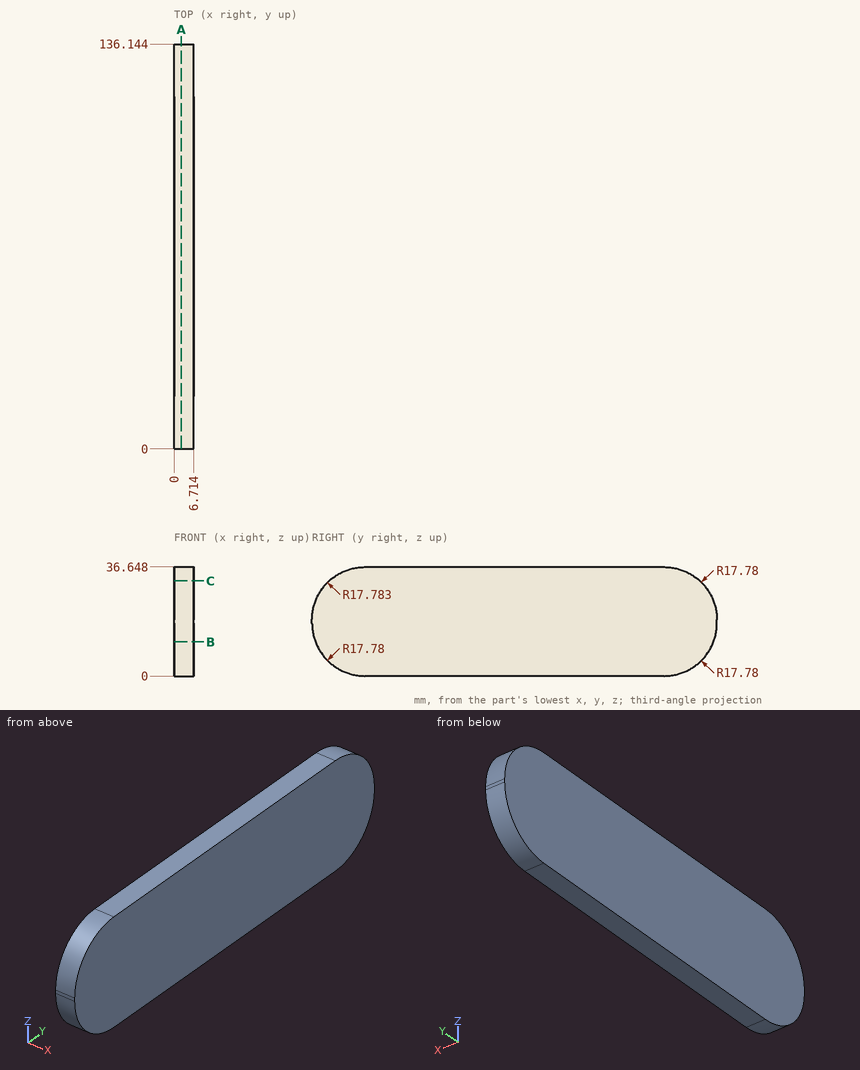
Input: dimensioned drawing with shaded views. Units: mm. Origin: part minimum x, y, z. Round coordinates to 2 decimals unless told otherwise and drop trailing zeros. Loops run counter-clockwise (first coordinate to the right, second up) from the corner with the lowest first, then second, coordinate; pieces in that order, holes last.
1) Pin query (flat end, axial travel): pin 1 (4 mm diameter, centred on x = 6, z = 10, fed in from -Y); pin 2 (1.5 mm diameter, centred on x = 4, z = 6.5, fed in from +Y); pin 3 (3 mm diameter, centred on x = 2, z = 30, fed in from +Y). Return the tip coordinate at first contact, or that it passes through.
Ans:
pin 1: stops at y = 0.97
pin 2: stops at y = 132.69
pin 3: stops at y = 133.31
2) Section query B-B on z = 11.5. Return the cut outline in (x, y), plus the area to 3 significant figures.
Ans:
outline: (0, 1.15) - (6.71, 1.15) - (6.71, 135) - (0, 135) - close
area: 899 mm2
3) Section query A-A on x = 2.5. Return the cut outline in (y, z) (3 decimals).
Ans:
outline: (0, 17.78) arc R17.78 ccw to (17.78, 0) - (118.364, 0) arc R17.78 ccw to (136.144, 17.78) - (136.144, 18.868) arc R17.78 ccw to (118.364, 36.648) - (17.783, 36.648) arc R17.783 ccw to (0, 18.865) - close
4) Material intervals for line 1 (Y direction, x = 4.25, z = 15.5); line 2 (Y direction, x = 1.25, z = 22); line 3 (Z direction, x = 2.75, y = 16.5), sorted ascending.
Ans:
line 1: y = 0.15 to 136
line 2: y = 0.28 to 135.87
line 3: z = 0.05 to 36.6
5) Section query C-C on z = 32. Return the cut outline in (x, y).
Ans:
outline: (0, 5.8) - (6.71, 5.8) - (6.71, 130.35) - (0, 130.35) - close
